The listing builds one solid part. Answer for the finished solid, in the listing's coordinates (mm). Face numbers are marked on the shaded views. A direction names the side the tool comes from. Give positions to 0.01 mm unless a question says otherwise; leave off trailing zeros. Write each loop counter-clockwise with the first axis right and the second up, starting at its lowest first coordinate (ties: lowest second). Pieces come first, ordered by that corner, then holes. Notation, with made-up numbers: (4.5, 2) -> (13.5, 2) arc R15 ccw to (13.5, 15) -> close; hole circle Ø6 at (-22.75, 0.5). An arc over 180 degrees is marked (long way). One line per question, with ' | ' between items.
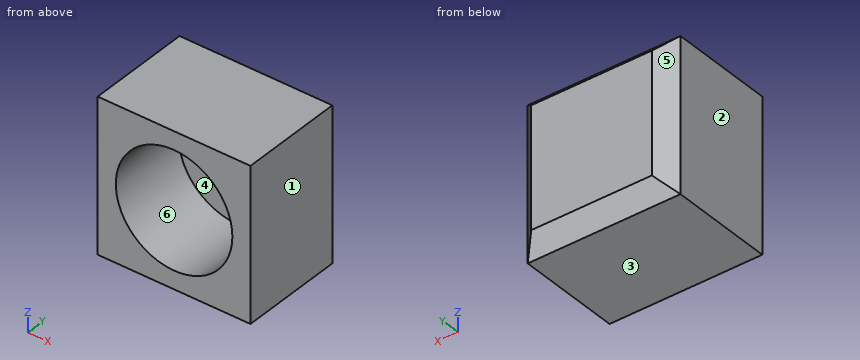
from build123d import *

# Parameters (mm, degrees)
SKETCH020_W       = 7.6
SKETCH020_H       = 7.6
PAD003_DEPTH      = 6
SKETCH022_R       = 2.8
PAD004_DEPTH      = 3
CYLINDER001_R     = 2.9
CYLINDER001_DEPTH = 10
CHAMFER_SIZE      = 0.8


with BuildPart() as part:
    # Sketch020 → Pad003 (new body)
    with BuildSketch(Plane.XZ):
        Rectangle(SKETCH020_W, SKETCH020_H)
    extrude(amount=PAD003_DEPTH)

    # Sketch022 → Pad004 (join)
    with BuildSketch(Plane.XZ.offset(6)):
        Circle(SKETCH022_R)
    extrude(amount=PAD004_DEPTH)

    # Cylinder001 → Cylinder001 (cut)
    with BuildSketch(Plane.XZ.offset(2)):
        Circle(CYLINDER001_R)
    extrude(amount=CYLINDER001_DEPTH, mode=Mode.SUBTRACT)

    # Chamfer
    chamfer_edges = [part.edges().sort_by_distance(p)[0] for p in [
        (3.8, 0, 0),
        (0, 0, -3.8),
        (0, 0, 3.8),
        (-3.8, 0, 0),
    ]]
    chamfer(chamfer_edges, length=CHAMFER_SIZE)


solid = part.part
Item 1: A flat-ended cylindrical pin translates along its axis: pin 1 (1.7 mm diameter, centred on x = 1, z = 0.5, fed in from -Y). Find the tip coordinate at first contact, or state that the pin passes through.
Answers below:
pin 1: y = -2
Item 2: Determine the mould class of the marked faces 1, 2, 3 and 4 for opening direction X: pulls with the +X half, pulls with the -X half, needs draft (parallel to the pull), parting line crosses it, or undercut.
Answers below:
face 1: pulls with the +X half | face 2: pulls with the -X half | face 3: needs draft | face 4: undercut
Item 3: Find section A-A (z = 2). Write down the section's boundary in (x, y).
Answers below:
outline: (-3.8, -6) -> (-2.1, -6) -> (-2.1, -2) -> (2.1, -2) -> (2.1, -6) -> (3.8, -6) -> (3.8, -0.8) -> (3, 0) -> (-3, 0) -> (-3.8, -0.8) -> close
Item 4: Find section D-D (z = 3.25). Write down the section's boundary in (x, y).
Answers below:
outline: (-3.8, -6) -> (3.8, -6) -> (3.8, -0.8) -> (3.25, -0.25) -> (-3.25, -0.25) -> (-3.8, -0.8) -> close
Item 5: Consider line 1 (Z direction, x = 0, y = -3.95); line 2 (Y direction, x = 2.25, z = 1.25). Determine where each line is inside the solid, lowest interval first. Write a range as [from, to].
Answers below:
line 1: [-3.8, -2.9], [2.9, 3.8] | line 2: [-2, 0]
Item 6: Find section B-B (y = -4.7). Write down the section's boundary in (x, z), then the cut area to 3 significant figures.
Answers below:
outline: (-3.8, -3.8) -> (3.8, -3.8) -> (3.8, 3.8) -> (-3.8, 3.8) -> close; hole circle Ø5.8 at (0, 0) | area: 31.3 mm²
Item 7: Find section C-C (x = 2). Write down the section's boundary in (y, z), then the cut area to 3 significant figures.
Answers below:
outline: (-6, -3.8) -> (-0.8, -3.8) -> (0, -3) -> (0, 3) -> (-0.8, 3.8) -> (-6, 3.8) -> (-6, 2.1) -> (-2, 2.1) -> (-2, -2.1) -> (-6, -2.1) -> close | area: 28.2 mm²
Item 8: A tool of negligible diameter and unlimited length cuts with its end or side. For the marked faces 5 and 6, from which of +Z, -Z, +X, -X, +Y, -Y can it reach the whole face along a straight path? Write none if from no direction.
Answers below:
face 5: +Z, -Z, -X, +Y | face 6: -Y
